The drawing under review shows one solid part. Ordinate dimensions are in mm from its lowest x, y, z. A direction names the side the tool comes from. Coordinates: 2 decimals unless noted, no trailing zeros. Write each loop counter-clockwise with the first axis right and the second up, starting at its lowest first coordinate (ties: lowest second). Pieces come first, ordered by that corner, then holes. Notation, with made-up numbers: (85.25, 23) -> (99.25, 23) arc R22 ccw to (99.25, 49) -> close; hole circle Ø11 at (-24, -25). An arc over 180 degrees is marked (long way). One line per item, written item: value. Start each with the question number.
1) Add section C-C (x = 28.5). State the section outline as (y, z) points (3 decimals).
2) Mouldability with a two-part tool opening along X and no side actions: class the marked faces 3, 4, 5 and 6 as released by +X, released by -X, zero draft, split by the parting line, or undercut.
3) For pin 1 Ø1.6 at (x, y) = (1, 14.5) entering from -Z; pin 2 Ø3.5 at (x, z) = (2, 182.5) entering from +Y (3 decimals); pin 3 Ø4 at (x, z) = (69.5, 126.5) entering from +Y (3 decimals), all flat-tipped, find the tip position at first contact; note any pin that passes through.
4) Add section D-D (z = 146). State the section outline as (x, y) points (3 decimals), and give its area (3 significant figures).
5) Add section B-B (z = 109.5). State the section outline as (x, y) points (3 decimals), and give its area (3 significant figures).
6) For probe 1 along X at (y, z) = (17, 34) (3 decimals); probe 2 along Y at (x, z) = (25, 101) (3 decimals); probe 3 along Z at (x, y) = (81.5, 17) (3 decimals), list the stretches that pass through material, from the lowest coordinate up. Write a range as from..to.
7) Machinability: for the marked faces 1 and 2, which of the approach directions +Z, -Z, +X, -X, +Y, -Y give a long, thin tool a straight path to every point of the face, cutting with its end or side? Answer none if there is none.
8) Add section A-A (y = 33). State the section outline as (x, z) points (3 decimals), and give its area (3 significant figures).
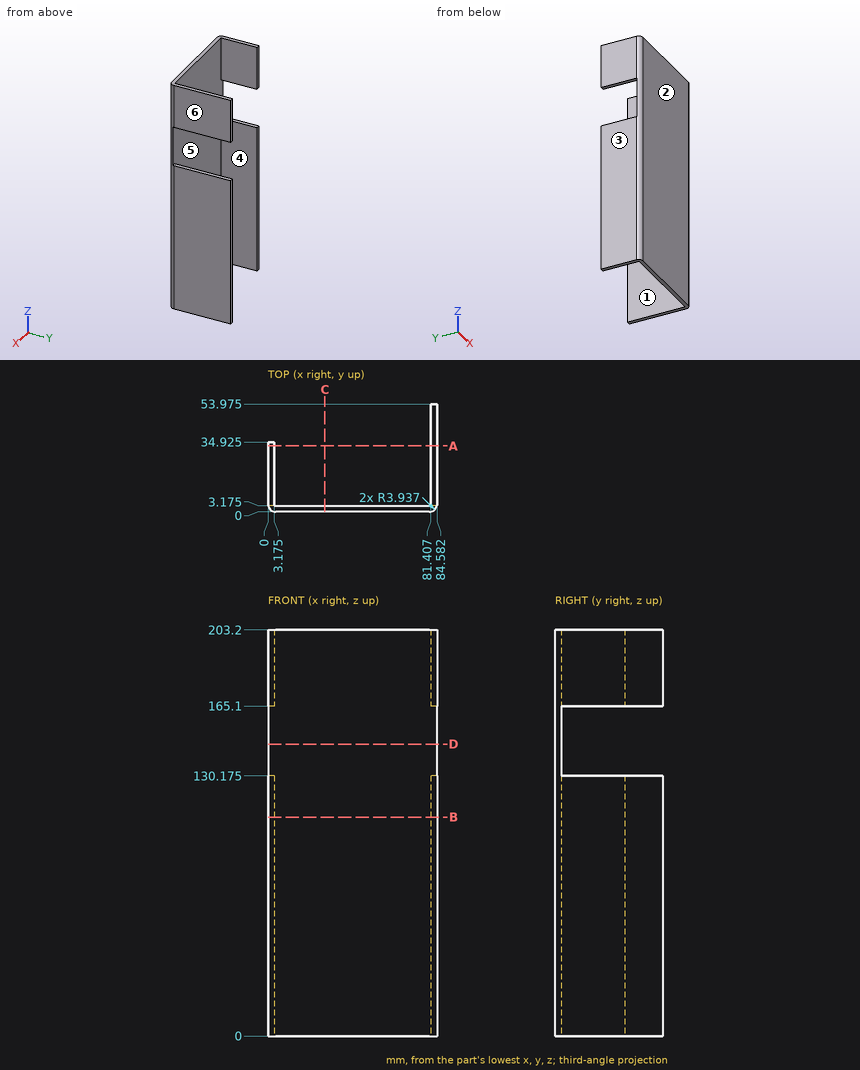
Numbers:
1. outline: (0, 0) -> (3.175, 0) -> (3.175, 203.2) -> (0, 203.2) -> close
2. face 3: released by -X
2. face 4: undercut
2. face 5: undercut
2. face 6: released by +X
3. pin 1: z = 0
3. pin 2: y = 34.925
3. pin 3: y = 3.175
4. outline: (0.074, 3.175) arc R3.937 ccw to (3.937, 0) -> (80.645, 0) arc R3.937 ccw to (84.508, 3.175) -> close
4. area: 262 mm²
5. outline: (0, 3.937) arc R3.937 ccw to (3.937, 0) -> (80.645, 0) arc R3.937 ccw to (84.582, 3.937) -> (84.582, 53.975) -> (81.407, 53.975) -> (81.407, 3.175) -> (3.175, 3.175) -> (3.175, 34.925) -> (0, 34.925) -> close
5. area: 524 mm²
6. probe 1: 0..3.175, 81.407..84.582
6. probe 2: 0..3.175
6. probe 3: 0..130.175, 165.1..203.2
7. face 1: +Z, -Z, +Y
7. face 2: +Z, -Z, +X, -X, -Y
8. outline: (0, 0) -> (3.175, 0) -> (3.175, 130.175) -> (0, 130.175) -> close; (0, 165.1) -> (3.175, 165.1) -> (3.175, 203.2) -> (0, 203.2) -> close; (81.407, 0) -> (84.582, 0) -> (84.582, 130.175) -> (81.407, 130.175) -> close; (81.407, 165.1) -> (84.582, 165.1) -> (84.582, 203.2) -> (81.407, 203.2) -> close
8. area: 1,070 mm²
